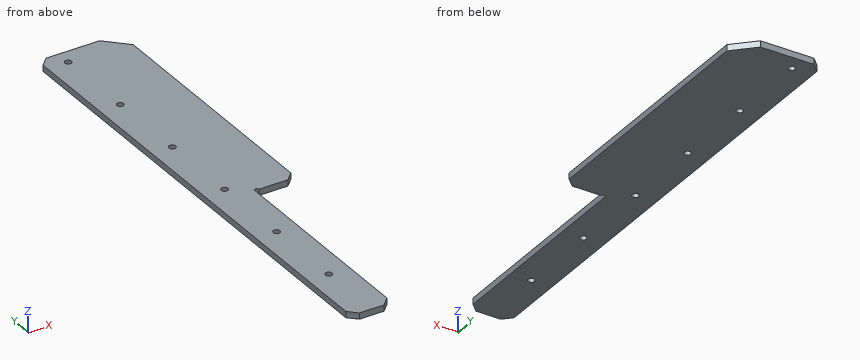
from build123d import *

# Parameters (mm, degrees)
EXTRUDE_1_DEPTH        = 1.5
SKETCH_2_R             = 1.6
CUT_EXTRUDE_1_DEPTH    = 137.506410106
PATTERN_LINEAR_1_COUNT = 6
PATTERN_LINEAR_1_PITCH = 40
CHAMFER_1_SIZE         = 10
CHAMFER_2_SIZE         = 4
SKETCH_3_R             = 1
CUT_EXTRUDE_2_DEPTH    = 137.506410106


with BuildPart() as part:
    # 草图1 → 凸台-拉伸1 (new, symmetric)
    with BuildSketch(Plane.XY):
        Polygon((-20, 135), (-20, -105.4), (0, -105.4), (0, 0), (20, 0), (20, 135), align=None)
    extrude(amount=EXTRUDE_1_DEPTH, both=True)

    # 草图2 → 切除-拉伸1 (cut, through all)
    with BuildSketch(Plane.XY.offset(1.5)):
        with Locations((-10, 127.5)):
            Circle(SKETCH_2_R)
    cut_extrude_1 = extrude(amount=-CUT_EXTRUDE_1_DEPTH, mode=Mode.SUBTRACT)

    # 阵列(线性)1: 切除-拉伸1 ×6
    with Locations(*[(0, -i * PATTERN_LINEAR_1_PITCH, 0) for i in range(1, PATTERN_LINEAR_1_COUNT)]):
        add(cut_extrude_1, mode=Mode.SUBTRACT)

    # 倒角1
    chamfer_1_edges = [part.edges().sort_by_distance(p)[0] for p in [
        (20, 135, 0),
    ]]
    chamfer(chamfer_1_edges, length=CHAMFER_1_SIZE)

    # 倒角2
    chamfer_2_edges = [part.edges().sort_by_distance(p)[0] for p in [
        (20, 0, 0),
        (0, -105.4, 0),
        (-20, -105.4, 0),
        (-20, 135, 0),
    ]]
    chamfer(chamfer_2_edges, length=CHAMFER_2_SIZE)

    # 草图3 → 切除-拉伸2 (cut, through all)
    with BuildSketch(Plane.XY.offset(1.5)):
        with Locations((1, 0)):
            Circle(SKETCH_3_R)
    extrude(amount=-CUT_EXTRUDE_2_DEPTH, mode=Mode.SUBTRACT)


solid = part.part
Geometry check sheet. Reference: the model listing, model coordinates, mm. Round coordinates to 2 decimals unless told otherwise and drop trailing zeros. Order: outer loops, then holes, each group sorted by start corner. A loop starts at its lowest first (then second) coordinate and runs counter-clockwise, first axis right, second up. Notation, with made-up numbers: M -35,18.25 L 18,18.25 A17 cw 18,42.25 Z; hole C 61.25,38.25 d10. An arc over 180 degrees is marked long. Answer in a Markdown table with one row per item. Add a question column.
Item 1: Depth check by flat-ended pin: pin 1 Ø2.5 at (x, y) = (-10, 127.5) entering from -Z; pin 2 Ø1.5 at (y, z) = (-65, 0) entering from +X; pin 3 Ø5 at (x, y) = (-10, 47.5) entering from -Z. Enter the tip coordinate at first touch or a pass-through.
Item 2: Material ranges on L1, parallel to X at y = 87.5, z = 0.05; L2, parallel to X at y = -88.5, z = 0.35; L3, parallel to Y at x = 1, z = 1, recorded low to high. Write a range as [from, to].
Item 3: Sectioned sample at A-A, the plane z = -0.6. Enter the section's corners in (x, y).
Filled in:
| question | item | result |
|---|---|---|
| 1 | pin 1 | passes through |
| 1 | pin 2 | stops at x = 0 |
| 1 | pin 3 | stops at z = -1.5 |
| 2 | L1 | x = [-20, -11.6], [-8.4, 20] |
| 2 | L2 | x = [-20, 0] |
| 2 | L3 | y = [1, 135] |
| 3 | outline | M -20,-101.4 L -16,-105.4 L -4,-105.4 L 0,-101.4 L 0,0 A1 cw 2,0 L 16,0 L 20,4 L 20,125 L 10,135 L -16,135 L -20,131 Z; hole C -10,-72.5 d3.2; hole C -10,-32.5 d3.2; hole C -10,7.5 d3.2; hole C -10,47.5 d3.2; hole C -10,87.5 d3.2; hole C -10,127.5 d3.2 |
